Autodesk Inventor part; units mm, degrees
ref_plane "YZ Plane" through (0, 0, 0) normal (1, 0, 0) x (0, 1, 0)
ref_plane "XZ Plane" through (0, 0, 0) normal (0, 1, 0) x (-1, 0, 0)
ref_plane "XY Plane" through (0, 0, 0) normal (0, 0, 1) x (1, 0, 0)
sketch "Sketch1" plane through (0, 0, 0) normal (0, 0, 1) x (1, 0, 0)
  arc A0 (0, 5) -> (0, -5) centre (0, 0) ccw
  line L0 (0, 0) -> (18, 0) construction
  line L1 (18, 5) -> (0, 5)
  line L2 (0, -5) -> (18, -5)
  arc A1 (18, -5) -> (18, 5) centre (18, 0) ccw
  dimension "d0" = 5
  dimension "d1" = 18
extrude "Extrusion1" add sketch "Sketch1" along normal blind 7
sketch "Sketch2" plane through (0, 0, 7) normal (0, 0, 1) x (1, 0, 0)
  arc A0 (18, -5) -> (18, 5) centre (18, 0) ccw
  arc A1 (0, 5) -> (0, -5) centre (0, 0) ccw
hole "Hole1" at (0, 0, 7) at (18, 0, 7) direction (0, 0, -1) diameter 4 end through all
sketch "Sketch3" plane through (0, 0, 7) normal (0, 0, 1) x (1, 0, 0)
  line L0 (0, 5) -> (18, 5)
  line L1 (18, -5) -> (0, -5)
  line L2 (12.5, 0.9) -> (5.5, 0.9)
  line L3 (5.5, 0.9) -> (5.5, -0.9)
  line L4 (5.5, -0.9) -> (12.5, -0.9)
  line L5 (12.5, -0.9) -> (12.5, 0.9)
  line L6 (12.5, -1.6) -> (5.5, -1.6)
  line L7 (5.5, -1.6) -> (5.5, -3.4)
  line L8 (5.5, -3.4) -> (12.5, -3.4)
  line L9 (12.5, -3.4) -> (12.5, -1.6)
  line L10 (12.5, 1.6) -> (5.5, 1.6)
  line L11 (5.5, 1.6) -> (5.5, 3.4)
  line L12 (5.5, 3.4) -> (12.5, 3.4)
  line L13 (12.5, 3.4) -> (12.5, 1.6)
  line L14 (5.5, 4.1) -> (12.5, 4.1)
  line L15 (12.5, 4.1) -> (12.5, 5)
  line L16 (12.5, 5) -> (5.5, 5)
  line L17 (5.5, 5) -> (5.5, 4.1)
  line L18 (12.5, -4.1) -> (5.5, -4.1)
  line L19 (5.5, -4.1) -> (5.5, -5)
  line L20 (5.5, -5) -> (12.5, -5)
  line L21 (12.5, -5) -> (12.5, -4.1)
  line L22 (9, 5) -> (9, -5) construction
  line L23 (9, 5) -> (9, 7.1624) construction
  line L24 (12.5, 3.4) -> (12.5, 4.1) construction
  line L25 (12.5, 1.6) -> (12.5, 0.9) construction
  line L26 (12.5, -0.9) -> (12.5, -1.6) construction
  line L27 (12.5, -3.4) -> (12.5, -4.1) construction
  point P0 (9, 4.1)
  dimension "d11" = 7
  dimension "d12" = 0.7
  dimension "d13" = 1.8
extrude "Extrusion2" cut sketch "Sketch3" against normal blind 0.5
properties part number "belt-clamp"
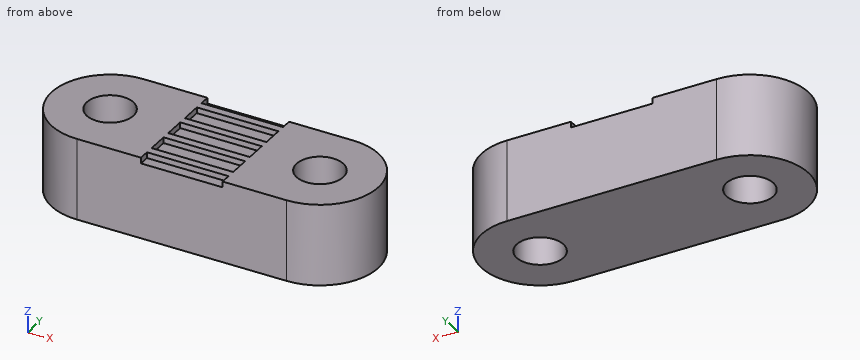
Part model, mm, in its own coordinate system. Round coordinates to 2 decimals unless told otherwise and drop trailing zeros. Write each loop counter-clockwise with the first axis right and the second up, starting at its lowest first coordinate (ties: lowest second). Pieces come first, ordered by that corner, then holes. Notation, with made-up numbers: (38, 68.5) -> (70, 68.5) arc R4 ccw to (70, 73.5) -> close; hole circle Ø4 at (80, -17.5). An arc over 180 degrees is marked (long way). Return JSON: item names as keys, results as strings. Group by question number.
Q1. Saw through at C-C on z = 4.75. Write the cut outline in (x, y).
Q2. Saw through at D-D on y = 3. Write the cut outline in (x, z), plus the area to 4 significant figures.
Q3. Probe L1, parallel to X at y = 0, z = 3.5; L2, parallel to Y at x = 18, z = 2.5; L3, parallel to X at y = -1.5, z = 5.75. List the from-to ranges inside material, lowest first. Write a range as [from, to].
Q4. Pin check, flat tips, straight feed: pin 1 (5 mm diameter, centred on x = 0.5, y = 3, fed in from -Z); pin 2 (2 mm diameter, centred on y = -1.5, z = 3, fed in from -X); pin 3 (2.5 mm diameter, centred on x = 18, y = 0, fed in from -Z); pin 4 (0.6 mm diameter, centred on x = 8, z = 7, fed in from -Y). Stop position of each tip, or through.
Q5. Saw through at A-A on y = 0. Write the cut outline in (x, z), plus the area to 4 significant figures.
Q6. Saw through at B-B on x = 18.75. Write the cut outline in (y, z).
Answer:
{
 "1": {"outline": "(0, -5) -> (18, -5) arc R5 ccw to (18, 5) -> (0, 5) arc R5 ccw to start; hole circle Ø4 at (0, 0); hole circle Ø4 at (18, 0)"},
 "2": {"outline": "(-4, 0) -> (22, 0) -> (22, 7) -> (12.5, 7) -> (12.5, 6.5) -> (5.5, 6.5) -> (5.5, 7) -> (-4, 7) -> close", "area": "178.5 mm2"},
 "3": {"L1": "[-5, -2], [2, 16], [20, 23]", "L2": "[-5, -2], [2, 5]", "L3": "[-4.77, -1.32], [1.32, 16.68], [19.32, 22.77]"},
 "4": {"pin 1": "z = 0", "pin 2": "x = -4.97", "pin 3": "through", "pin 4": "y = -4.1"},
 "5": {"outline": "(-5, 0) -> (-2, 0) -> (-2, 7) -> (-5, 7) -> close; (2, 0) -> (16, 0) -> (16, 7) -> (12.5, 7) -> (12.5, 6.5) -> (5.5, 6.5) -> (5.5, 7) -> (2, 7) -> close; (20, 0) -> (23, 0) -> (23, 7) -> (20, 7) -> close", "area": "136.5 mm2"},
 "6": {"outline": "(-4.94, 0) -> (-1.85, 0) -> (-1.85, 7) -> (-4.94, 7) -> close; (1.85, 0) -> (4.94, 0) -> (4.94, 7) -> (1.85, 7) -> close"}
}
